from build123d import *

# Parameters (mm, degrees)
F0_W     = 600
F0_H     = 20
F1_DEPTH = 600
F2_W     = 55
F2_H     = 26
F3_DEPTH = 28.5
F4_R     = 8
F5_DEPTH = 26


with BuildPart() as f1:
    # F0 (on Front) → F1 (new body)
    with BuildSketch(Plane.XZ):
        with Locations((-2.310631, 10)):
            Rectangle(F0_W, F0_H)
    extrude(amount=F1_DEPTH)

    # F2 (on face) → F3 (join)
    with BuildSketch(Plane.XY.offset(20)):
        with Locations((270.189369, -13)):
            Rectangle(F2_W, F2_H)
    extrude(amount=F3_DEPTH)

    # F4 (on face) → F5 (cut, through all)
    with BuildSketch(Plane.XZ.offset(26)):
        with Locations((270.189369, 34.000836)):
            Circle(F4_R)
    extrude(amount=-F5_DEPTH, mode=Mode.SUBTRACT)


solid = f1.part
CAD build for the part. Positions are in the model's coordinates, mm. A direction names the side the tool comes from. Round coordinates to 2 decimals unless told otherwise and drop trailing zeros. Loops run counter-clockwise (first coordinate to the right, second up) from the corner with the lowest first, then second, coordinate; pieces in that order, holes last.
(1) Drop flat-ended pins along their axis: pin 1 (8.5 mm diameter, centred on x = 284, z = 34, fed in from -Y); pin 2 (1.5 mm diameter, centred on x = -178.5, y = -528, fed in from +Z); pin 3 (8 mm diameter, centred on y = -16.5, z = 38, fed in from -X). Give the stop position or say it passes through.
(2) Which spindle directions (+Z, -Z, +X, -X, +Y, -Y) get a long thin tool onto all of the face, cutting with end or side? Do faces 1 (the flat face through (264, -26, 28)), 2 (the flat face through (-7, 0, 13)), 3 (the flat face through (242.689, -13, 34)). Say none if no direction does.
(3) Cut at A-A (x = 164). Give the cut face in (y, z).
(4) Wall check: line 1 along Z through (x, y) = (-21.5, -491). Give the ranges that are in metal, low to high.
(5) Two-plate mould, pull along X, no slides. Class faces 4 (the cylindrical face through (277.82, -13.18, 36.4)), 5 (the flat face through (-302.311, -296, 10)), 6 (the flat face through (-7, -296, 20)): +X half, -X half, draft (parallel to the pull), parting line (faces both ways), or undercut.
(6) Cut at B-B (y = -88). Give the cut face in (x, z), plus the area to 3 significant figures.
Findings below:
1. pin 1: stops at y = -26
1. pin 2: stops at z = 20
1. pin 3: stops at x = 242.69
2. face 1: +Z, +X, -X, -Y
2. face 2: +Z, -Z, +X, -X, +Y
2. face 3: +Z, -X, +Y, -Y
3. outline: (-600, 0) - (0, 0) - (0, 20) - (-600, 20) - close
4. line 1: z = 0 to 20
5. face 4: undercut
5. face 5: -X half
5. face 6: draft
6. outline: (-302.31, 0) - (297.69, 0) - (297.69, 20) - (-302.31, 20) - close
6. area: 12,000 mm2
